```python
from build123d import *

# Parameters (mm, degrees)
EXTRUDE_1_DEPTH = 3
FILLET_1_R      = 0.5
FILLET_2_R      = 1


with BuildPart() as part:
    # Эскиз1 → Бобышка-Вытянуть1 (new body)
    with BuildSketch(Plane.XY):
        Polygon((3, 0), (0, 0), (0, 3), (8, 3), (16, -5), (16, -13), (13, -13), (13, -10), (3, -10), align=None)
        Polygon((3, 8), (3, 3), (8, 3), align=None)
        Polygon((21, -10), (16, -5), (16, -10), align=None)
    extrude(amount=EXTRUDE_1_DEPTH)

    # Скругление1
    fillet_1_edges = [part.edges().sort_by_distance(p)[0] for p in [
        (0, 0, 1.5),
        (0, 3, 1.5),
        (16, -13, 1.5),
        (13, -13, 1.5),
    ]]
    fillet(fillet_1_edges, radius=FILLET_1_R)

    # Скругление2
    fillet_2_edges = [part.edges().sort_by_distance(p)[0] for p in [
        (3, -10, 1.5),
    ]]
    fillet(fillet_2_edges, radius=FILLET_2_R)


solid = part.part
```
Check sheet for the modelled part. Datum: model origin and axes. Units: mm. A direction names the side the tool comes from. Round coordinates to 2 decimals unless told otherwise and drop trailing zeros. Order: outer loops, then holes, each group sorted by start corner. A loop starts at its lowest first (then second) coordinate and runs counter-clockwise, first axis right, second up.
1) Go/stop test with flat-tipped pins: pin 1 Ø0.8 at (y, z) = (-11.5, 2) entering from +X; pin 2 Ø1.5 at (y, z) = (-9.5, 2) entering from -X; pin 3 Ø1.5 at (x, z) = (8, 1.5) entering from +Y. Record where each tip stops, or that it passes through.
2) Tool access check on faces 1 (the flat face through (15, -13, 1)), 2 (the flat face through (3, 6, 1)), 3 (the flat face through (16, -11, 1)), 4 (the flat face through (8, -5, 0)), 5 (the flat face through (3, -5, 1)). Record the directions out of +Z, -Z, +X, -X, +Y, -Y that give a thin tool (end or side, any length) a straight path to the whole face; none if there is none.
3) Scan lines: line 1 (Y direction, x = 7, z = 2.5); line 2 (X direction, y = -11.5, z = 1.95); line 3 (X direction, y = -7, z = 1.5). Record each from-to range of solid material in increasing order.
4) Section check B-B (x = 12.75). Record the boundary of the cut face in (y, z), and give its area (4 significant figures).
5) Section check A-A (z = 2.6). Record the boundary of the cut face in (x, y), and give its area (3 significant figures).
6) Section check C-C (y = 4.75). Record the boundary of the cut face in (x, z), and give its area (3 significant figures).
Result:
1. pin 1: stops at x = 16
1. pin 2: stops at x = 3
1. pin 3: stops at y = 3.75
2. face 1: +Z, -Z, +X, -X, -Y
2. face 2: +Z, -Z, -X, +Y
2. face 3: +Z, -Z, +X, -Y
2. face 4: -Z, +X, -X, +Y, -Y
2. face 5: +Z, -Z, -X, -Y
3. line 1: y = -10 to 4
3. line 2: x = 13 to 16
3. line 3: x = 3 to 18
4. outline: (-10, 0) - (-1.75, 0) - (-1.75, 3) - (-10, 3) - close
4. area: 24.75 mm2
5. outline: (0, 0.5) arc R0.5 ccw to (0.5, 0) - (3, 0) - (3, -9) arc R1 ccw to (4, -10) - (13, -10) - (13, -12.5) arc R0.5 ccw to (13.5, -13) - (15.5, -13) arc R0.5 ccw to (16, -12.5) - (16, -10) - (21, -10) - (3, 8) - (3, 3) - (0.5, 3) arc R0.5 ccw to (0, 2.5) - close
5. area: 180 mm2
6. outline: (3, 0) - (6.25, 0) - (6.25, 3) - (3, 3) - close
6. area: 9.75 mm2
